Work out the finished part from the listing and answer in its coordinate system (mm). Face numbers are marked on the shaded views. A direction names the side the tool comes from. Round coordinates to 2 decimals unless told otherwise and drop trailing zeros. Loops run counter-clockwise (first coordinate to the right, second up) from the corner with the lowest first, then second, coordinate; pieces in that order, holes last.
from build123d import *

# Parameters (mm, degrees)
BOX124_W               = 12
BOX124_H               = 44
BOX124_DEPTH           = 10
BOX119_W               = 4
BOX119_H               = 1
BOX119_DEPTH           = 7
BOX127_W               = 4
BOX127_H               = 1
BOX127_DEPTH           = 7
BOX128_W               = 4
BOX128_H               = 2
BOX128_DEPTH           = 7
BOX130_W               = 4
BOX130_H               = 1
BOX130_DEPTH           = 7
BOX122_W               = 4
BOX122_H               = 1
BOX122_DEPTH           = 7
BOX121_W               = 4
BOX121_H               = 7.2
BOX121_DEPTH           = 7
BOX120_W               = 13
BOX120_H               = 40
BOX120_DEPTH           = 10
BOX120_PITCH_ANGLE     = -45
BOX123_W               = 10
BOX123_H               = 2
BOX123_DEPTH           = 7
BOX126_W               = 10
BOX126_H               = 2
BOX126_DEPTH           = 7
BOX125_W               = 10
BOX125_H               = 2
BOX125_DEPTH           = 7
BOX129_W               = 10
BOX129_H               = 2
BOX129_DEPTH           = 7
BOX131_W               = 5
BOX131_H               = 40
BOX131_DEPTH           = 7
CHAMFER011_SIZE        = 4
CUT034_PLACEMENT_ANGLE = 180
CUT033_PLACEMENT_ANGLE = 180


with BuildPart() as cube108:
    # Box124 → Box124 (new body)
    with BuildSketch(Plane(origin=(-11, -2, -12), x_dir=(1, 0, 0), z_dir=(0, 0, 1))):
        with Locations((6, 22)):
            Rectangle(BOX124_W, BOX124_H)
    extrude(amount=BOX124_DEPTH)


with BuildPart() as cube103:
    # Box119 → Box119 (new body)
    with BuildSketch(Plane(origin=(-1, 12, 0), x_dir=(1, 0, 0), z_dir=(0, 0, 1))):
        with Locations((2, 0.5)):
            Rectangle(BOX119_W, BOX119_H)
    extrude(amount=BOX119_DEPTH)


with BuildPart() as cube111:
    # Box127 → Box127 (new body)
    with BuildSketch(Plane(origin=(-1, 36.6, 0), x_dir=(1, 0, 0), z_dir=(0, 0, 1))):
        with Locations((2, 0.5)):
            Rectangle(BOX127_W, BOX127_H)
    extrude(amount=BOX127_DEPTH)


with BuildPart() as cube112:
    # Box128 → Box128 (new body)
    with BuildSketch(Plane(origin=(-1, 8, 0), x_dir=(1, 0, 0), z_dir=(0, 0, 1))):
        with Locations((2, 1)):
            Rectangle(BOX128_W, BOX128_H)
    extrude(amount=BOX128_DEPTH)


with BuildPart() as cube114:
    # Box130 → Box130 (new body)
    with BuildSketch(Plane(origin=(-1, 24.4, 0), x_dir=(1, 0, 0), z_dir=(0, 0, 1))):
        with Locations((2, 0.5)):
            Rectangle(BOX130_W, BOX130_H)
    extrude(amount=BOX130_DEPTH)


with BuildPart() as cube106:
    # Box122 → Box122 (new body)
    with BuildSketch(Plane(origin=(-1, 5, 0), x_dir=(1, 0, 0), z_dir=(0, 0, 1))):
        with Locations((2, 0.5)):
            Rectangle(BOX122_W, BOX122_H)
    extrude(amount=BOX122_DEPTH)


with BuildPart() as fusion038:
    # Box121 → Box121 (new body)
    with BuildSketch(Plane(origin=(-1, 27.4, 0), x_dir=(1, 0, 0), z_dir=(0, 0, 1))):
        with Locations((2, 3.6)):
            Rectangle(BOX121_W, BOX121_H)
    extrude(amount=BOX121_DEPTH)

    # Fusion038: union Cube103, Cube111, Cube112, Cube114, Cube106
    add(cube103.part)
    add(cube111.part)
    add(cube112.part)
    add(cube114.part)
    add(cube106.part)


with BuildPart() as sphere044:
    # Sphere044 → Sphere044 (revolve)
    with BuildSketch(Plane(origin=(-3, 28, 2.5), x_dir=(1, 0, 0), z_dir=(0, -1, 0))):
        with BuildLine():
            ThreePointArc((0, -1.5), (1.5, 0), (0, 1.5))
            Line((0, 1.5), (0, -1.5))
        make_face()
    revolve(axis=Axis((-3, 28, 2.5), (0, 0, 1)))


with BuildPart() as fusion040:
    # Sphere046 → Sphere046 (revolve)
    with BuildSketch(Plane(origin=(-3, 34, 2.5), x_dir=(1, 0, 0), z_dir=(0, -1, 0))):
        with BuildLine():
            ThreePointArc((0, -1.5), (1.5, 0), (0, 1.5))
            Line((0, 1.5), (0, -1.5))
        make_face()
    revolve(axis=Axis((-3, 34, 2.5), (0, 0, 1)))

    # Fusion040: union Sphere044
    add(sphere044.part)


with BuildPart() as sphere045:
    # Sphere045 → Sphere045 (revolve)
    with BuildSketch(Plane(origin=(-3, 11.5, 2.5), x_dir=(1, 0, 0), z_dir=(0, -1, 0))):
        with BuildLine():
            ThreePointArc((0, -1.25), (1.25, 0), (0, 1.25))
            Line((0, 1.25), (0, -1.25))
        make_face()
    revolve(axis=Axis((-3, 11.5, 2.5), (0, 0, 1)))


with BuildPart() as cube104:
    # Box120 → Box120 (new body)
    with BuildSketch(Plane.XY):
        with Locations((6.5, 20)):
            Rectangle(BOX120_W, BOX120_H)
    extrude(amount=BOX120_DEPTH)


with BuildPart() as cube104_1:
    # Box120 pitch: moved
    add(cube104.part.rotate(Axis((0, 0, 0), (0, 1, 0)), BOX120_PITCH_ANGLE))


with BuildPart() as cube104_2:
    # Box120 placement: moved
    add(cube104_1.part.moved(Location((-10.19, 0, -1.19))))


with BuildPart() as cube107:
    # Box123 → Box123 (new body)
    with BuildSketch(Plane(origin=(-10, 6, 0), x_dir=(1, 0, 0), z_dir=(0, 0, 1))):
        with Locations((5, 1)):
            Rectangle(BOX123_W, BOX123_H)
    extrude(amount=BOX123_DEPTH)


with BuildPart() as cube110:
    # Box126 → Box126 (new body)
    with BuildSketch(Plane(origin=(-10, 10, 0), x_dir=(1, 0, 0), z_dir=(0, 0, 1))):
        with Locations((5, 1)):
            Rectangle(BOX126_W, BOX126_H)
    extrude(amount=BOX126_DEPTH)


with BuildPart() as cube109:
    # Box125 → Box125 (new body)
    with BuildSketch(Plane(origin=(-10, 25.4, 0), x_dir=(1, 0, 0), z_dir=(0, 0, 1))):
        with Locations((5, 1)):
            Rectangle(BOX125_W, BOX125_H)
    extrude(amount=BOX125_DEPTH)


with BuildPart() as cube113:
    # Box129 → Box129 (new body)
    with BuildSketch(Plane(origin=(-10, 34.6, 0), x_dir=(1, 0, 0), z_dir=(0, 0, 1))):
        with Locations((5, 1)):
            Rectangle(BOX129_W, BOX129_H)
    extrude(amount=BOX129_DEPTH)


with BuildPart() as cut035:
    # Box131 → Box131 (new body)
    with BuildSketch(Plane.XY):
        with Locations((2.5, 20)):
            Rectangle(BOX131_W, BOX131_H)
    extrude(amount=BOX131_DEPTH)

    # Fusion041: union Cube107, Cube110, Cube109, Cube113
    add(cube107.part)
    add(cube110.part)
    add(cube109.part)
    add(cube113.part)

    # Cut035: cut Cube104
    add(cube104_2.part, mode=Mode.SUBTRACT)


with BuildPart() as cut033:
    # Sphere043 → Sphere043 (revolve)
    with BuildSketch(Plane(origin=(-3, 6.5, 2.5), x_dir=(1, 0, 0), z_dir=(0, -1, 0))):
        with BuildLine():
            ThreePointArc((0, -1.25), (1.25, 0), (0, 1.25))
            Line((0, 1.25), (0, -1.25))
        make_face()
    revolve(axis=Axis((-3, 6.5, 2.5), (0, 0, 1)))

    # Fusion039: union Sphere045, Cut035
    add(sphere045.part)
    add(cut035.part)

    # Cut036: cut Fusion040
    add(fusion040.part, mode=Mode.SUBTRACT)

    # Chamfer011
    chamfer011_edges = [cut033.edges().sort_by_distance(p)[0] for p in [
        (-9, 7, 0),
        (-9, 11, 0),
        (-9, 35.6, 0),
        (-9, 26.4, 0),
    ]]
    chamfer(chamfer011_edges, length=CHAMFER011_SIZE)

    # Cut034: cut Fusion038
    add(fusion038.part, mode=Mode.SUBTRACT)


with BuildPart() as cut033_1:
    # Cut034 placement: moved
    add(cut033.part.moved(Location((-5, 40, 3))).rotate(Axis((-5, 40, 3), (1, 0, 0)), CUT034_PLACEMENT_ANGLE))

    # Cut033: cut Cube108
    add(cube108.part, mode=Mode.SUBTRACT)


with BuildPart() as cut033_2:
    # Cut033 placement: moved
    add(cut033_1.part.moved(Location((40, 40, 0))).rotate(Axis((40, 40, 0), (0, 0, 1)), CUT033_PLACEMENT_ANGLE))


solid = cut033_2.part
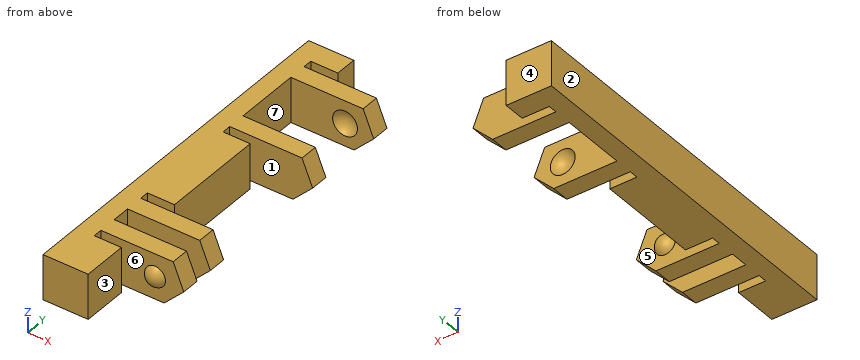
Item 1: Section D-D, the plane z = 2.45 is taken. Give the vertices of the cut face in (x, y), plus the area to 3 significant figures.
Item 2: Straight lines are drawn through the part: line 1 (Y direction, x = 49.25, z = 2.5); line 2 (Y direction, x = 49, z = 0.8); line 3 (X direction, y = 22, z = 2.65). For each, find the intervals that lie inside material, in ascending order.
Item 3: Each of these flat-tipped pins is pushed along its axis until it touches: P1, Ø2, axis at x = 45.5, z = 1.5, coming from the -Y side; P2, Ø1, axis at x = 48, z = -0.5, coming from the +Y side; P3, Ø1.1, axis at y = 24.5, z = 0.5, coming from the +X side; P4, Ø1.5, axis at y = 12.5, z = 1, coming from the +X side. Where does it stop, or does it pass through?
Item 4: Section A-A, the plane x = 43.25 is taken. Give the vertices of the cut face in (y, z).
Item 5: For the marked faces 1, 2 and 3, determine the directions among +Z, -Z, +X, -X, +Y, -Y from which every point of the face is accessible in a straight line to the end or side of a thin tool.
Item 6: Section C-C, the plane y = 31.5 is taken. Give the vertices of the cut face in (x, z).
Item 7: Section B-B, the plane z = -1.6 is taken. Give the vertices of the cut face in (x, y), plus the area to 3 significant figures.
Item 8: Determine the mould class of the marked faces 4, 5, 6 and 7 for opening direction X: pulls with the +X half, pulls with the -X half, needs draft (parallel to the pull), parting line crosses it, or undercut.
Answer below:
1. outline: (40, 0) - (45, 0) - (45, 5) - (42, 5) - (42, 6) - (50.23, 6) - (50.23, 8) - (42, 8) - (42, 10) - (50.23, 10) - (50.23, 12) - (42, 12) - (42, 13) - (45, 13) - (45, 24.4) - (42, 24.4) - (42, 25.4) - (50.23, 25.4) - (50.23, 27.4) - (42, 27.4) - (42, 34.6) - (50.23, 34.6) - (50.23, 36.6) - (42, 36.6) - (42, 37.6) - (45, 37.6) - (45, 40) - (40, 40) - close
1. area: 202 mm2
2. line 1: y = 6 to 8, 10 to 12, 25.4 to 27.4, 34.6 to 36.6
2. line 2: y = 5.81 to 8, 10 to 12.19, 25.4 to 26.92, 35.08 to 36.6
2. line 3: x = 40 to 45
3. P1: stops at y = 0
3. P2: stops at y = 36.6
3. P3: stops at x = 45
3. P4: stops at x = 51.06
4. outline: (0, -2) - (5, -2) - (5, 3) - (0, 3) - close; (6, -2) - (8, -2) - (8, 3) - (6, 3) - close; (10, -2) - (12, -2) - (12, 3) - (10, 3) - close; (13, -2) - (24.4, -2) - (24.4, 3) - (13, 3) - close; (25.4, -2) - (27.4, -2) - (27.4, 3) - (25.4, 3) - close; (34.6, -2) - (36.6, -2) - (36.6, 3) - (34.6, 3) - close; (37.6, -2) - (40, -2) - (40, 3) - (37.6, 3) - close
5. face 1: +Z, -Z, +X
5. face 2: +Z, -Z, -X, +Y, -Y
5. face 3: +Z, -Z, +X, -Y
6. outline: (40, -2) - (42, -2) - (42, 3) - (40, 3) - close
7. outline: (40, 0) - (45, 0) - (45, 5) - (42, 5) - (42, 6) - (49.4, 6) - (49.4, 8) - (42, 8) - (42, 10) - (49.4, 10) - (49.4, 12) - (42, 12) - (42, 13) - (45, 13) - (45, 24.4) - (42, 24.4) - (42, 25.4) - (49.4, 25.4) - (49.4, 27.4) - (42, 27.4) - (42, 34.6) - (49.4, 34.6) - (49.4, 36.6) - (42, 36.6) - (42, 37.6) - (45, 37.6) - (45, 40) - (40, 40) - close
7. area: 196 mm2
8. face 4: needs draft
8. face 5: undercut
8. face 6: undercut
8. face 7: pulls with the +X half
